from build123d import *

# Parameters (mm, degrees)
SKETCH_1_R          = 1.5
EXTRUDE_1_DEPTH     = 5
EXTRUDE_2_DEPTH     = 3
EXTRUDE_START       = -1.5
SKETCH_3_R          = 2.5
EXTRUDE_3_DEPTH     = 3
CUT_EXTRUDE_START   = -1.5
SKETCH_4_R          = 1
CUT_EXTRUDE_1_DEPTH = 3
EXTRUDE_4_DEPTH     = 3
EXTRUDE_5_DEPTH     = 3
SKETCH_9_R          = 1
EXTRUDE_6_DEPTH     = 3
EXTRUDE_7_DEPTH     = 3
EXTRUDE_START_2     = 1.5
EXTRUDE_8_DEPTH     = 3
CHAMFER_5_SIZE      = 0.25
CHAMFER_6_SIZE      = 0.25


with BuildPart() as part:
    # 草图1 → 凸台-拉伸1 (new body)
    with BuildSketch(Plane(origin=(0, 0, 0), x_dir=(1, 0, 0), z_dir=(0, 1, 0))):
        with Locations(Location((0, 0, 0), (0, 0, 270))):
            Circle(SKETCH_1_R)
    extrude(amount=EXTRUDE_1_DEPTH)

    # 草图2 → 凸台-拉伸2 (add)
    with BuildSketch(Plane(origin=(0, 0, 0), x_dir=(1, 0, 0), z_dir=(0, 1, 0))):
        with BuildLine():
            Line((50, 1.5), (50, -1.5))
            Line((50, -1.5), (2.598076211, -1.5))
            ThreePointArc((2.598076211, -1.5), (-3, 0), (2.598076211, 1.5))
            Line((2.598076211, 1.5), (50, 1.5))
        make_face()
    extrude(amount=-EXTRUDE_2_DEPTH)

    # 草图3 → 凸台-拉伸3 (add)
    with BuildSketch(Plane.XY.offset(EXTRUDE_START)):
        with Locations((50, -1.5)):
            Circle(SKETCH_3_R)
    extrude(amount=EXTRUDE_3_DEPTH)

    # 草图4 → 切除-拉伸1 (cut)
    with BuildSketch(Plane.XY.offset(CUT_EXTRUDE_START)):
        with Locations(Location((50, -1.5, 0), (0, 0, 180))):
            Circle(SKETCH_4_R)
    extrude(amount=CUT_EXTRUDE_1_DEPTH, mode=Mode.SUBTRACT)

    # 草图5 → 凸台-拉伸4 (add)
    with BuildSketch(Plane(origin=(0, 0, 0), x_dir=(1, 0, 0), z_dir=(0, 1, 0))):
        with BuildLine():
            Line((5.098076211, 1.5), (0.925764755, 2.853587149))
            ThreePointArc((0.925764755, 2.853587149), (1.88743565, 2.331863347), (2.598076211, 1.5))
            Line((2.598076211, 1.5), (5.098076211, 1.5))
        make_face()
        with BuildLine():
            Line((5.098076211, -1.5), (0.925764755, -2.853587149))
            ThreePointArc((0.925764755, -2.853587149), (1.88743565, -2.331863347), (2.598076211, -1.5))
            Line((2.598076211, -1.5), (5.098076211, -1.5))
        make_face()
    extrude(amount=-EXTRUDE_4_DEPTH)

    # 草图6 → 凸台-拉伸5 (add)
    with BuildSketch(Plane.XY.offset(EXTRUDE_START)):
        with BuildLine():
            Line((45.5, 0), (49.421854812, 0.932231104))
            ThreePointArc((49.421854812, 0.932231104), (48.629244055, 0.590700395), (48, 0))
            Line((48, 0), (45.5, 0))
        make_face()
        with BuildLine():
            Line((45.5, -3), (49.421854812, -3.932231104))
            ThreePointArc((49.421854812, -3.932231104), (48.629244055, -3.590700395), (48, -3))
            Line((48, -3), (45.5, -3))
        make_face()
    extrude(amount=EXTRUDE_5_DEPTH)

    # 草图9 → 凸台-拉伸6 (add)
    with BuildSketch(Plane.XY.offset(EXTRUDE_START)):
        with BuildLine():
            Line((16.621216129, 0), (34.913425822, 15.348986407))
            ThreePointArc((34.913425822, 15.348986407), (37.396444401, 19.390597315), (32.985062993, 17.647119736))
            Line((32.985062993, 17.647119736), (11.954044649, 0))
            Line((11.954044649, 0), (16.621216129, 0))
        make_face()
        with Locations(Location((35.481333294, 17.783628291, 0), (0, 0, 180))):
            Circle(SKETCH_9_R, mode=Mode.SUBTRACT)
    extrude(amount=EXTRUDE_6_DEPTH)

    # 草图10 → 凸台-拉伸7 (add)
    with BuildSketch(Plane.XY.offset(EXTRUDE_START)):
        with BuildLine():
            Line((32.998314714, 13.742017382), (36.601856403, 15.548806606))
            ThreePointArc((36.601856403, 15.548806606), (35.775149629, 15.300953934), (34.913425822, 15.348986407))
            Line((34.913425822, 15.348986407), (32.998314714, 13.742017382))
        make_face()
        with BuildLine():
            Line((31.069951885, 16.040150712), (33.475040368, 19.275200849))
            ThreePointArc((33.475040368, 19.275200849), (33.08739701, 18.504092773), (32.985062993, 17.647119736))
            Line((32.985062993, 17.647119736), (31.069951885, 16.040150712))
        make_face()
    extrude(amount=EXTRUDE_7_DEPTH)

    # 草图11 → 凸台-拉伸8 (add)
    with BuildSketch(Plane.XY.offset(EXTRUDE_START_2)):
        Polygon((31.045694114, 12.103574157), (35.451034835, 0), (32.443670675, 0), (28.741919511, 10.170477737), align=None)
    extrude(amount=-EXTRUDE_8_DEPTH)

    # 倒角5
    chamfer_5_edges = [part.edges().sort_by_distance(p)[0] for p in [
        (37.396444401, 19.390597315, 1.5),
        (32.272496126, 17.65767578, -1.5),
        (32.272496126, 17.65767578, 1.5),
        (22.68156782, 5.085238868, 1.5),
        (22.68156782, 5.085238868, -1.5),
        (40.475517418, 0, 1.5),
        (24.532443402, 0, -1.5),
        (30.592795093, 5.085238868, 1.5),
        (33.248364474, 6.051787078, 1.5),
        (30.592795093, 5.085238868, -1.5),
        (33.248364474, 6.051787078, -1.5),
        (51, -1.5, -1.5),
        (51, -1.5, 1.5),
        (8.52606043, 0, 1.5),
        (25.299038106, -3, 1.5),
        (25.299038106, -3, -1.5),
        (47.460927406, -3.466115552, -1.5),
        (47.460927406, -3.466115552, 1.5),
        (52.5, -1.5, -1.5),
        (52.5, -1.5, 1.5),
        (40.475517418, 0, -1.5),
        (47.460927406, 0.466115552, -1.5),
        (47.460927406, 0.466115552, 1.5),
        (8.52606043, 0, -1.5),
        (24.532443402, 0, 1.5),
        (21.511998267, 8.020075356, 1.5),
        (21.511998267, 8.020075356, -1.5),
        (36.481333294, 17.783628291, 1.5),
        (32.022004414, 12.92279577, 1.5),
        (32.022004414, 12.92279577, -1.5),
        (34.800085558, 14.645411994, -1.5),
        (34.800085558, 14.645411994, 1.5),
        (37.396444401, 19.390597315, -1.5),
    ]]
    chamfer(chamfer_5_edges, length=CHAMFER_5_SIZE)

    # 倒角6
    chamfer_6_edges = [part.edges().sort_by_distance(p)[0] for p in [
        (3.397221816, 0, -2.051793575),
        (3.397221816, 0, 2.051793575),
        (-3, 0, 0),
        (3.397221816, -3, -2.051793575),
        (3.397221816, -3, 2.051793575),
        (-3, -3, 0),
    ]]
    chamfer(chamfer_6_edges, length=CHAMFER_6_SIZE)


solid = part.part
Can you work these out from the model? Positions are in its coordinate system, mm. A direction names the side the tool comes from. Round coordinates to 2 decimals unless told otherwise and drop trailing zeros. Loops run counter-clockwise (first coordinate to the right, second up) from the corner with the lowest first, then second, coordinate; pieces in that order, holes last. Notation, with made-up numbers: (9, 87) - (52, 87) arc R19 ccw to (52, 123) - close; hole circle Ø2 at (-21.75, 20). An arc over 180 degrees is marked (long way). Write item = value, one per line. Start each with the question number.
(1) If we mould it in two halves opening along Y, with no side actions, what happens to faces 6 (the face through (47.45, -3.34, -1.37)), 7 (the face through (32.008, 12.911, -0.018)), 8 (the face through (47.5, 0.35, -1.37)), 9 (the face through (30.736, 5.052, -1.373))? For each: released by +Y, released by -Y, zero draft, split by the parting line, or undercut.
(2) If we section it at B-B (y = -1.5): Please give me the cut outline in (x, z).
(3) If I drill on probe 1 along Y at (x, z) = (50, 0.4); probe 2 along Y at (x, z) = (18.5, 1.35); probe 3 along Y at (x, z) = (44, -0.55), over which ranges is the centre line in solid material (lowest first)? Write a range as [from, to].
(4) If we section it at A-A (x = 50): Please give me the cut outline in (y, z), and give its area (3 significant figures).
(5) For faces 1 (the face through (22.597, 5.014, -0.017)), 2 (the face through (34.77, 14.63, -0.02)), 3 (the face through (21.7, 8.02, -1.37)), 4 (the face through (29, -1, -1.5)), 5 (the face through (22.39, 5, -1.37)), which set-ups out of +Z, -Z, +X, -X, +Y, -Y let a thin tool reach every point of the face, with its end or its side?
(6) If we section it at D-D (x = 7): Please give me the cut outline in (y, z), and give its area (4 significant figures).
(7) For P1, Ø2.5, axis at x = 35.48, y = 17.78, coming from the -Z side; P2, Ø0.8, axis at x = 39, z = 0, coming from the +Y side; P3, Ø7, axis at x = 28.5, y = 5, coming from the +Z side, each with a flat end and sliding along its axis, tell me the tip position at first contact or that it passes through.
(8) If we section it at C-C (z = 0): Please give me the cut outline in (x, y), and give its area (3 significant figures).
Ans:
q1.face_6 = released by -Y
q1.face_7 = undercut
q1.face_8 = released by +Y
q1.face_9 = undercut
q2.outline = (0.93, -2.85) - (5.1, -1.5) - (48.75, -1.5) - (49, -1.25) - (49, 1.25) - (48.75, 1.5) - (5.1, 1.5) - (0.93, 2.85) arc R3 ccw (long way) to start; (51, -1.25) - (51.25, -1.5) - (52.25, -1.5) - (52.5, -1.25) - (52.5, 1.25) - (52.25, 1.5) - (51.25, 1.5) - (51, 1.25) - close
q3.probe_1 = [-4, -2.5], [-0.5, 1]
q3.probe_2 = [-2.9, -0.1], [1.71, 5.36]
q3.probe_3 = [-3, 0]
q4.outline = (-4, -1.25) - (-3.75, -1.5) - (-2.75, -1.5) - (-2.5, -1.25) - (-2.5, 1.25) - (-2.75, 1.5) - (-3.75, 1.5) - (-4, 1.25) - close; (-0.5, -1.25) - (-0.25, -1.5) - (0.75, -1.5) - (1, -1.25) - (1, 1.25) - (0.75, 1.5) - (-0.25, 1.5) - (-0.5, 1.25) - close
q4.area = 8.75 mm²
q5.face_1 = +Z, -Z
q5.face_2 = +Z, -Z, +X
q5.face_3 = -Z, +Y
q5.face_4 = -Z, +X, +Y, -Y
q5.face_5 = -Z
q6.outline = (-3, -1.25) - (-2.75, -1.5) - (-0.25, -1.5) - (0, -1.25) - (0, 1.25) - (-0.25, 1.5) - (-2.75, 1.5) - (-3, 1.25) - close
q6.area = 8.875 mm²
q7.P1 = -1.5
q7.P2 = 0
q7.P3 = 1.5
q8.outline = (-3, -2.75) - (-2.75, -3) - (45.5, -3) - (49.42, -3.93) arc R2.5 ccw (long way) to (49.42, 0.93) - (45.5, 0) - (35.45, 0) - (31.05, 12.1) - (33, 13.74) - (36.6, 15.55) arc R2.5 ccw (long way) to (33.48, 19.28) - (31.07, 16.04) - (11.95, 0) - (1.5, 0) - (1.5, 5) - (-1.5, 5) - (-1.5, 0) - (-2.75, 0) - (-3, -0.25) - close; hole (16.62, 0) - (32.44, 0) - (28.74, 10.17) - close; hole circle Ø2 at (35.48, 17.78); hole circle Ø2 at (50, -1.5)
q8.area = 313 mm²
